Here's how the part is built. I have some questions about the finished solid (model axes, mm). A direction names the side the tool comes from. Coordinates: 2 decimals unless noted, no trailing zeros. Loops run counter-clockwise (first coordinate to the right, second up) from the corner with the lowest first, then second, coordinate; pieces in that order, holes last. Notation, with made-up numbers: (-4, 78.5) -> (2, 78.5) arc R31 cw to (2, 111.5) -> close; hole circle Ø8 at (-3.75, 22). An arc over 180 degrees is marked (long way). Use CSV: the item, a comma, the result in double quotes. Start each with the question number.
from build123d import *

# Parameters (mm, degrees)
F1_DEPTH = 20
F2_W     = 3.5
F2_H     = 3
F3_DEPTH = 78
F4_W     = 3.5
F4_H     = 3
F5_DEPTH = 78
F6_W     = 3.5
F6_H     = 3
F7_DEPTH = 78


with BuildPart() as f1:
    # F0 (on Top) → F1 (new body)
    with BuildSketch(Plane.XY):
        with BuildLine():
            Line((58.5386705788, 35.5735020327), (12.3347873053, 7.4957558301))
            Line((12.3347873053, 7.4957558301), (25.3178172443, -13.8687224833))
            Line((25.3178172443, -13.8687224833), (93.6841478472, 27.6769733213))
            Line((93.6841478472, 27.6769733213), (80.7011179083, 49.0414516348))
            Line((80.7011179083, 49.0414516348), (71.3573575668, 43.3633199961))
            ThreePointArc((71.3573575668, 43.3633199961), (72.1702047448, 41.4907764357), (72.4480140728, 39.4684110144))
            ThreePointArc((72.4480140728, 39.4684110144), (66.9703794941, 32.2462203424), (58.5386705788, 35.5735020327))
        make_face()
        with BuildLine():
            Line((-0.6482426336, 28.8602341436), (12.3347873053, 7.4957558301))
            Line((12.3347873053, 7.4957558301), (58.5386705788, 35.5735020327))
            ThreePointArc((58.5386705788, 35.5735020327), (61.0531050911, 45.8777545084), (71.3573575668, 43.3633199961))
            Line((71.3573575668, 43.3633199961), (80.7011179083, 49.0414516348))
            Line((80.7011179083, 49.0414516348), (67.7180879693, 70.4059299482))
            Line((67.7180879693, 70.4059299482), (-0.6482426336, 28.8602341436))
        make_face()
        with BuildLine():
            Line((-24.6695746107, -14.9915116603), (-12.6589086221, 6.9343612416))
            Line((-12.6589086221, 6.9343612416), (-60.0813298697, 32.9116559437))
            ThreePointArc((-60.0813298697, 32.9116559437), (-70.1179765686, 30.1888598259), (-73.2270059229, 40.1126611203))
            Line((-73.2270059229, 40.1126611203), (-82.8217019083, 45.368492405))
            Line((-82.8217019083, 45.368492405), (-94.8323678969, 23.4426195031))
            Line((-94.8323678969, 23.4426195031), (-24.6695746107, -14.9915116603))
        make_face()
        with BuildLine():
            Line((1.5386516322, -68.5018912218), (0.3241213168, -14.4301170718))
            Line((0.3241213168, -14.4301170718), (-24.6695746107, -14.9915116603))
            Line((-24.6695746107, -14.9915116603), (-22.8731119275, -94.9713386283))
            Line((-22.8731119275, -94.9713386283), (2.120584, -94.4099440398))
            Line((2.120584, -94.4099440398), (1.8754883853, -83.4981087782))
            ThreePointArc((1.8754883853, -83.4981087782), (-5.7910387695, -76.1684183766), (1.5386516322, -68.5018912218))
        make_face()
        with BuildLine():
            Line((25.3178172443, -13.8687224833), (0.3241213168, -14.4301170718))
            Line((0.3241213168, -14.4301170718), (1.5386516322, -68.5018912218))
            ThreePointArc((1.5386516322, -68.5018912218), (6.950487891, -70.6374848334), (9.2070700088, -76))
            ThreePointArc((9.2070700088, -76), (7.0695851754, -81.2434178823), (1.8754883853, -83.4981087782))
            Line((1.8754883853, -83.4981087782), (2.120584, -94.4099440398))
            Line((2.120584, -94.4099440398), (27.1142799275, -93.8485494513))
            Line((27.1142799275, -93.8485494513), (25.3178172443, -13.8687224833))
        make_face()
        with BuildLine():
            Line((-60.0813298697, 32.9116559437), (-12.6589086221, 6.9343612416))
            Line((-12.6589086221, 6.9343612416), (-0.6482426336, 28.8602341436))
            Line((-0.6482426336, 28.8602341436), (-70.8110359198, 67.2943653069))
            Line((-70.8110359198, 67.2943653069), (-82.8217019083, 45.368492405))
            Line((-82.8217019083, 45.368492405), (-73.2270059229, 40.1126611203))
            ThreePointArc((-73.2270059229, 40.1126611203), (-64.7960153912, 44.0670230084), (-59.014776772, 36.7666216964))
            ThreePointArc((-59.014776772, 36.7666216964), (-59.2863311657, 34.7667281702), (-60.0813298697, 32.9116559437))
        make_face()
        with BuildLine():
            Line((0.3241213168, -14.4301170718), (0.2245578354, -9.997478371))
            ThreePointArc((0.2245578354, -9.997478371), (-8.5457913254, -5.1932119756), (-8.7703491608, 4.8042663954))
            Line((-8.7703491608, 4.8042663954), (-12.6589086221, 6.9343612416))
            Line((-12.6589086221, 6.9343612416), (-24.6695746107, -14.9915116603))
            Line((-24.6695746107, -14.9915116603), (0.3241213168, -14.4301170718))
        make_face()
        with BuildLine():
            ThreePointArc((-8.7703491608, 4.8042663954), (-0.2245578354, 9.997478371), (8.5457913254, 5.1932119756))
            Line((8.5457913254, 5.1932119756), (12.3347873053, 7.4957558301))
            Line((12.3347873053, 7.4957558301), (-0.6482426336, 28.8602341436))
            Line((-0.6482426336, 28.8602341436), (-12.6589086221, 6.9343612416))
            Line((-12.6589086221, 6.9343612416), (-8.7703491608, 4.8042663954))
        make_face()
        with BuildLine():
            ThreePointArc((8.5457913254, 5.1932119756), (9.6295875627, 2.6964872284), (10, 0))
            ThreePointArc((10, 0), (7.1500202221, -6.991223843), (0.2245578354, -9.997478371))
            Line((0.2245578354, -9.997478371), (0.3241213168, -14.4301170718))
            Line((0.3241213168, -14.4301170718), (25.3178172443, -13.8687224833))
            Line((25.3178172443, -13.8687224833), (12.3347873053, 7.4957558301))
            Line((12.3347873053, 7.4957558301), (8.5457913254, 5.1932119756))
        make_face()
    extrude(amount=F1_DEPTH)

    # F2 (on face) → F3 (cut)
    with BuildSketch(Plane(origin=(-82.8217019083, 45.368492405, 0), x_dir=(-0.4804266395, -0.8770349161, 0), z_dir=(-0.8770349161, 0.4804266395, 0))):
        with Locations((23.25, 18.5)):
            Rectangle(F2_W, F2_H)
        with Locations((23.25, 1.5)):
            Rectangle(F2_W, F2_H)
    extrude(amount=-F3_DEPTH, mode=Mode.SUBTRACT)

    # F4 (on face) → F5 (cut)
    with BuildSketch(Plane(origin=(2.120584, -94.4099440398, 0), x_dir=(0.9997478371, 0.0224557835, 0), z_dir=(0.0224557835, -0.9997478371, 0))):
        with Locations((23.25, 18.5)):
            Rectangle(F4_W, F4_H)
        with Locations((23.25, 1.5)):
            Rectangle(F4_W, F4_H)
    extrude(amount=-F5_DEPTH, mode=Mode.SUBTRACT)

    # F6 (on face) → F7 (cut)
    with BuildSketch(Plane(origin=(80.7011179083, 49.0414516348, 0), x_dir=(-0.5193211976, 0.8545791325, 0), z_dir=(0.8545791325, 0.5193211976, 0))):
        with Locations((23.25, 18.5)):
            Rectangle(F6_W, F6_H)
        with Locations((23.25, 1.5)):
            Rectangle(F6_W, F6_H)
    extrude(amount=-F7_DEPTH, mode=Mode.SUBTRACT)


solid = f1.part
1) I want a section at B-B, the plane x = -65. Please give me the cut outline in (y, z), plus the area to 3 significant figures.
2) I want a section at C-C, the plane y = 17. Please give me the cut outline in (x, z), plus the area to 3 significant figures.
3) Thinking about a two-plate mould opening in X: for faces 1 (the face through (36.674, 47.445, 18.479)), 2 (the face through (-60, 7, 3)), 3 (the face through (-59.43, 8.04, 1.48)), which applies, pulls with the +X half, pulls with the -X half, needs draft (parallel to the pull), parting line crosses it, or undercut?
4) I want a section at D-D, the plane y = -56.5. Please give me the cut outline in (x, z).
5) For P1, Ø12, axis at x = -20, z = 11, coming from the -Y side; P2, Ø6, axis at y = -76, z = 4.5, coming from the -X side; P3, Ø6, axis at x = 33.5, z = 9.5, coming from the -Y side, each with a flat end and sliding along its axis, tell me the tip position at first contact or that it passes through.
6) I want a section at A-A, the plane z = 6.75. Please give me the cut outline in (x, y), plus the area to 3 significant figures.
7) Which directions (+Z, -Z, +X, -X, +Y, -Y) give clear straight access to the entire face, cutting with the end or side of a thin tool? Please do faces 4 (the face through (34.01, 49.92, 9.86)), 5 (the face through (24, -55, 3)), 6 (the face through (36.674, 47.445, 1.479)), 7 (the face through (36, 49, 17)).
8) Please list where these lines run through material, in increasing order: L1, parallel to Y at x = 5.5, z = 10; L2, parallel to X at y = 42.5, z = 2.5; L3, parallel to Z at x = 18, y = 37.5. Write a range as [from, to].
Return value:
1,outline,"(7.1, 3) -> (11.09, 3) -> (11.09, 0) -> (29.42, 0) -> (29.42, 20) -> (11.09, 20) -> (11.09, 17) -> (7.1, 17) -> close; (44.11, 0) -> (64.11, 0) -> (64.11, 20) -> (44.11, 20) -> close"
1,area,"822 mm²"
2,outline,"(-83.07, 3) -> (-75.79, 3) -> (-75.79, 0) -> (76.11, 0) -> (76.11, 20) -> (-75.79, 20) -> (-75.79, 17) -> (-83.07, 17) -> close"
2,area,"3,140 mm²"
3,face 1,"undercut"
3,face 2,"needs draft"
3,face 3,"pulls with the -X half"
4,outline,"(-23.74, 0) -> (22.77, 0) -> (22.77, 3) -> (26.28, 3) -> (26.28, 17) -> (22.77, 17) -> (22.77, 20) -> (-23.74, 20) -> close"
5,P1,"stops at y = -94.97"
5,P2,"stops at x = -23.37"
5,P3,"stops at y = -10.72"
6,outline,"(-94.83, 23.44) -> (-24.67, -14.99) -> (-22.87, -94.97) -> (27.11, -93.85) -> (25.32, -13.87) -> (93.68, 27.68) -> (67.72, 70.41) -> (-0.65, 28.86) -> (-70.81, 67.29) -> close; hole circle Ø15 at (-66.51, 36.77); hole circle Ø20 at (0, 0); hole circle Ø15 at (1.71, -76); hole circle Ø15 at (64.95, 39.47)"
6,area,"12,200 mm²"
7,face 4,"+Z, -Z, +Y"
7,face 5,"-Z, +X"
7,face 6,"-Z, +Y"
7,face 7,"+Z, +Y"
8,L1,"y = [-94.33, -82.47], [-69.53, -8.35], [8.35, 32.6]"
8,L2,"x = [-84.39, -71.35], [-61.68, -25.55], [28.54, 58.09], [71.81, 84.68]"
8,L3,"z = [3, 17]"
